Build history of the part. All positions in model axes, mm. A direction names the side the tool comes from. Round coordinates to 2 decimals unless told otherwise and drop trailing zeros. Write each loop counter-clockwise with the first axis right and the second up, starting at its lowest first coordinate (ties: lowest second). Pieces come first, ordered by that corner, then holes.
1) Which spindle directions (+Z, -Z, +X, -X, +Y, -Y) get a long thin tool onto all of the face, cutting with end or side? Do faces 4 (the cylindrical face through (-16.436, 8.741, 2.535)), 5 (the cylindrical face through (0, -5, 3)), 6 (the cylindrical face through (-17, 0, 1)). Say none if no direction does.
2) Flat gauge pins, fed straight in: pin 1 (1.6 mm diameter, centred on x = 12.45, y = 0, fed in from -Z); pin 2 (1.1 mm diameter, centred on x = 6.45, y = 0, fed in from +Z); pin 3 (1 mm diameter, centred on x = 10.5, z = 1.5, fed in from +Y); pin 4 (1.5 mm diameter, centred on x = 14.5, z = 4.5, fed in from +Y). Where does each tip first touch, or does it go through?
3) Wall check: probe 1 along Y at (x, z) = (-6.5, 2.7); probe 2 along Y at (x, z) = (8, 4.8); probe 3 along Y at (x, z) = (-7.5, 4.5). Give the ranges that are in metal, low to high.
4) Pull direction X, two halves, no side cores. Call faces 1 (the flat face through (-9.63, 2.55, 1.23)), 2 (the cylindrical face through (16.241, -8.936, 2.535)), 3 (the flat face through (0, 12.5, 2)): +X half, -X half, draft (parallel to the pull), parting line (faces both ways), or undercut.
5) Saw through at B-B (x = 0). Write the cut outline in (y, z), plus the area to 3 significant figures.
6) Saw through at C-C (y = -6.5). Write the cut outline in (x, z).
7) Saw through at A-A (z = 0.85). State how many separate pieces and enclosed holes the cut face has, plus the area to 3 significant figures.
from build123d import *

# Parameters (mm, degrees)
SKETCH1_W              = 40
SKETCH1_H              = 25
BOSS_EXTRUDE2_DEPTH    = 5
CUT_EXTRUDE1_DEPTH     = 2.5
CUT_EXTRUDE2_START     = -2.5
CUT_EXTRUDE2_OUTLINE_R = 0.6
CUT_EXTRUDE2_DEPTH     = 2.5
SKETCH7_R              = 5
CUT_EXTRUDE3_DEPTH     = 25.109126902
SKETCH8_R              = 2.5
CUT_EXTRUDE4_DEPTH     = 25.109126902
FILLET1_R              = 12.5


# Read off the part's stored shape, not the designer's step: Cut-Extrude2
with BuildPart() as part:
    # Sketch1 → Boss-Extrude2 (new body)
    with BuildSketch(Plane.XY):
        Rectangle(SKETCH1_W, SKETCH1_H)
    extrude(amount=BOSS_EXTRUDE2_DEPTH)

    # Sketch4 → Cut-Extrude1 (cut)
    with BuildSketch(Plane(origin=(0, 0, 0), x_dir=(-1, 0, 0), z_dir=(0, 0, -1))):
        with BuildLine():
            Line((-0.35, 3.48245603), (-15.2, 1.989974874))
            ThreePointArc((-15.2, 1.989974874), (-17, 0), (-15.2, -1.989974874))
            Line((-15.2, -1.989974874), (-0.35, -3.48245603))
            ThreePointArc((-0.35, -3.48245603), (0, -3.5), (0.35, -3.48245603))
            Line((0.35, -3.48245603), (15.2, -1.989974874))
            ThreePointArc((15.2, -1.989974874), (17, 0), (15.2, 1.989974874))
            Line((15.2, 1.989974874), (0.35, 3.48245603))
            ThreePointArc((0.35, 3.48245603), (0, 3.5), (-0.35, 3.48245603))
        make_face()
    extrude(amount=-CUT_EXTRUDE1_DEPTH, mode=Mode.SUBTRACT)

    # Cut-Extrude2 outline → Cut-Extrude2 (cut)
    with BuildSketch(Plane(origin=(0, 0, 2.5), x_dir=(-1, 0, 0), z_dir=(0, 0, -1)).offset(CUT_EXTRUDE2_START)):
        with BuildLine():
            ThreePointArc((3.982303371, 0.375845531), (4, 0), (3.982303371, -0.375845531))
            ThreePointArc((3.982303371, -0.375845531), (5.05, 0), (3.982303371, 0.375845531))
        make_face()
        with Locations((-4.45, 0)):
            Circle(CUT_EXTRUDE2_OUTLINE_R)
        with Locations((-6.45, 0)):
            Circle(CUT_EXTRUDE2_OUTLINE_R)
        with Locations((-8.45, 0)):
            Circle(CUT_EXTRUDE2_OUTLINE_R)
        with Locations((-14.45, 0)):
            Circle(CUT_EXTRUDE2_OUTLINE_R)
        with Locations((8.45, 0)):
            Circle(CUT_EXTRUDE2_OUTLINE_R)
        with Locations((10.45, 0)):
            Circle(CUT_EXTRUDE2_OUTLINE_R)
        with Locations((12.45, 0)):
            Circle(CUT_EXTRUDE2_OUTLINE_R)
        with Locations((14.45, 0)):
            Circle(CUT_EXTRUDE2_OUTLINE_R)
        with Locations((-12.45, 0)):
            Circle(CUT_EXTRUDE2_OUTLINE_R)
        with Locations((-10.45, 0)):
            Circle(CUT_EXTRUDE2_OUTLINE_R)
        with Locations((6.45, 0)):
            Circle(CUT_EXTRUDE2_OUTLINE_R)
    extrude(amount=CUT_EXTRUDE2_DEPTH, mode=Mode.SUBTRACT)

    # Sketch7 → Cut-Extrude3 (cut, through all)
    with BuildSketch(Plane(origin=(0, 0, 0), x_dir=(-1, 0, 0), z_dir=(0, 0, -1))):
        Circle(SKETCH7_R)
    extrude(amount=-CUT_EXTRUDE3_DEPTH, mode=Mode.SUBTRACT)

    # Sketch8 → Cut-Extrude4 (cut, through all)
    with BuildSketch(Plane.XY.offset(5)):
        with Locations((6.5, 6.5)):
            Circle(SKETCH8_R)
        with Locations((-6.5, 6.5)):
            Circle(SKETCH8_R)
        with Locations((-6.5, -6.5)):
            Circle(SKETCH8_R)
        with Locations((6.5, -6.5)):
            Circle(SKETCH8_R)
    extrude(amount=-CUT_EXTRUDE4_DEPTH, mode=Mode.SUBTRACT)

    # Fillet1
    fillet1_edges = [part.edges().sort_by_distance(p)[0] for p in [
        (-20, 12.5, 2.5),
        (-20, -12.5, 2.5),
        (20, -12.5, 2.5),
        (20, 12.5, 2.5),
    ]]
    fillet(fillet1_edges, radius=FILLET1_R - 0.0001)  # a hair under: the kernel refuses the full size


solid = part.part
Evaluation:
1. face 4: +Z, -Z, -X, +Y
1. face 5: +Z, -Z
1. face 6: -Z
2. pin 1: stops at z = 2.5
2. pin 2: passes through
2. pin 3: stops at y = 12.25
2. pin 4: stops at y = 10.83
3. probe 1: y = -12.5 to -9, -4 to -0.6, 0.6 to 4, 9 to 12.5
3. probe 2: y = -12.49 to -8.5, -4.5 to -0.4, 0.4 to 4.5, 8.5 to 12.49
3. probe 3: y = -12.5 to -8.79, -4.21 to 4.21, 8.79 to 12.5
4. face 1: undercut
4. face 2: +X half
4. face 3: draft
5. outline: (-12.5, 0) - (-5, 0) - (-5, 5) - (-12.5, 5) - close; (5, 0) - (12.5, 0) - (12.5, 5) - (5, 5) - close
5. area: 75.0 mm2
6. outline: (-18.18, 0) - (-9, 0) - (-9, 5) - (-18.18, 5) - close; (-4, 0) - (4, 0) - (4, 5) - (-4, 5) - close; (9, 0) - (18.18, 0) - (18.18, 5) - (9, 5) - close
7. separate pieces: 1
7. enclosed holes: 5
7. area: 592 mm2
